from build123d import *

# Parameters (mm, degrees)
SKETCH1_R           = 2.6375
BOSS_EXTRUDE1_DEPTH = 4


with BuildPart() as part:
    # Sketch1 → Boss-Extrude1 (new body)
    with BuildSketch(Plane.XY.offset(4)):
        with BuildLine():
            Line((46.037988185, 74.138222759), (26.891590001, 77.042584155))
            ThreePointArc((26.891590001, 77.042584155), (22.54509271, 75.572516008), (21.227396241, 71.177426126))
            Line((21.227396241, 71.177426126), (23.568249259, 58.696629092))
            ThreePointArc((23.568249259, 58.696629092), (26.381296021, 55.081304051), (30.958043521, 55.274150009))
            Line((30.958043521, 55.274150009), (47.763588686, 64.850585648))
            ThreePointArc((47.763588686, 64.850585648), (50.20397723, 70.108121575), (46.037988185, 74.138222759))
        make_face()
        with Locations((45.288105172, 69.194775028)):
            Circle(SKETCH1_R, mode=Mode.SUBTRACT)
        with Locations((26.141706988, 72.099136424)):
            Circle(SKETCH1_R, mode=Mode.SUBTRACT)
        with Locations((28.482560007, 59.618339389)):
            Circle(SKETCH1_R, mode=Mode.SUBTRACT)
    extrude(amount=-BOSS_EXTRUDE1_DEPTH)


solid = part.part
Geometry: final body of the model. Coordinates: model frame, mm. Round coordinates to 2 decimals unless told otherwise and drop trailing zeros. Loops run counter-clockwise (first coordinate to the right, second up) from the corner with the lowest first, then second, coordinate; pieces in that order, holes last. Notation, with made-up numbers: M -4.75,82.25 L 47.25,82.25 A15 cw 47.25,101.25 Z; hole C 23.25,22.5 d5. An arc over 180 degrees is marked long. Put each result on its own line as item: value. Start each with the question number.
(1) Section query C-C (z = 0.4). Return loops of the section in (x, y) (1 decimal).
(2) Contact query for flat-ended pins moving along their axis: pin 1 Ø2 at (y, z) = (61, 3.5) entering from -X; pin 2 Ø1.5 at (x, z) = (33, 1.5) entering from -Y; pin 3 Ø1.5 at (x, z) = (46, 1.5) entering from -Y; pin 4 Ø4.5 at (x, y) = (45.29, 69.19) entering from +Z. Output: stop coordinate, or through.
(3) Material intervals for line 1 along X through (y, z) = (71.5, 1.15); line 2 along Y through (x, z) = (26.75, 0.8); line 3 along X through (y, z) = (72, 3.7), sorted ascending. Write a range as [from, to].
(4) Draft query along Y for faces 1 (the face through (36, 66, 0)), 2 (the face through (26.32, 55.11, 2.03)), 3 (the face through (29.7, 57.28, 2.03)). Return one class per face: +Y half, -Y half, draft (parallel to the pull), parting line (faces both ways), or undercut.
(5) Section query D-D (x = 37.25). Return loops of the section in (y, z), then the cut area to 3 significant figures.
(6) Section query A-A (y = 57.5). Return loops of the section in (x, z).
(7) Section query B-B (x = 44). Return loops of the section in (y, z).
Findings below:
1. outline: M 21.2,71.2 L 23.6,58.7 A5 ccw 31,55.3 L 47.8,64.9 A5 ccw 46,74.1 L 26.9,77 A5 ccw Z; hole C 26.1,72.1 d5.3; hole C 28.5,59.6 d5.3; hole C 45.3,69.2 d5.3
2. pin 1: stops at x = 22.95
2. pin 2: stops at y = 56.01
2. pin 3: stops at y = 63.42
2. pin 4: passes through
3. line 1: x = [21.18, 23.57], [28.71, 44.01], [46.57, 49.72]
3. line 2: y = [54.93, 57.63], [61.61, 69.53], [74.67, 77.06]
3. line 3: x = [21.14, 23.51], [28.78, 49.43]
4. face 1: draft
4. face 2: -Y half
4. face 3: undercut
5. outline: M 58.86,0 L 75.47,0 L 75.47,4 L 58.86,4 Z
5. area: 66.4 mm2
6. outline: M 23.95,0 L 26.91,0 L 26.91,4 L 23.95,4 Z; M 30.05,0 L 34.86,0 L 34.86,4 L 30.05,4 Z
7. outline: M 62.71,0 L 66.89,0 L 66.89,4 L 62.71,4 Z; M 71.5,0 L 74.45,0 L 74.45,4 L 71.5,4 Z
